CAD build for the part. Positions are in the model's coordinates, mm. Coordinates: 2 decimals unless noted, no trailing zeros. Loops run counter-clockwise (first coordinate to the right, second up) from the corner with the lowest first, then second, coordinate; pieces in that order, holes last. Notation, with made-up numbers: (70, 52.5) -> (103, 52.5) arc R38 ccw to (103, 91.5) -> close; hole circle Ø10 at (60.25, 56). An arc over 180 degrees is marked (long way). Return JSON: item names as keys, results as strings. Group by question number.
(1) Saw through at C-C on y = -2.5. Write the cut outline in (x, z).
(2) Probe L1, parallel to X at y = 6.5, z = 0; L2, parallel to X at y = 11.25, z = 3.5; L3, parallel to Z at x = 4, y = -5.75. List the from-to ranges inside material, lowest first.
(3) Flat gauge pins, fed straight in: pin 1 Ø3 at (y, z) = (5, 3.5) entering from -X; pin 2 Ø2 at (y, z) = (-4, -4) entering from -X. Where does each tip first touch, or does it go through?
(4) Mould opens along X. For faces 1 (the face through (-1.352, 0.182, 4.292)), 2 (the face through (0.1, -0.17, 6.35)), 3 (the face through (-4, -13, -3)) say: pulls with the +X half, pulls with the -X half, needs draft (parallel to the pull), parting line crosses it, or undercut.
(5) Saw through at B-B on x = 0. Write the cut outline in (y, z).
(6) Saw through at A-A on z = 0. Write the cut outline in (x, y).
```python
from build123d import *

# Parameters (mm, degrees)
CUT_EXTRUDE1_DEPTH      = 16.800158227
CUT_EXTRUDE1_DEPTH_BACK = 16.800158227
SKETCH2_W               = 6.200894729
SKETCH2_H               = 5
SKETCH2_W_2             = 7.80745867


with BuildPart() as part:
    # Sketch1 → Revolve1 (revolve)
    with BuildSketch(Plane.XY, mode=Mode.PRIVATE) as revolve1_sk:
        Polygon((-4.5, 13), (-5.35, 13), (-6.35, 12), (-6.35, -12), (-5.35, -13), (-4.5, -13), align=None)
    revolve(revolve1_sk.sketch.rotate(Axis((0, 18.016627358, 0), (0, -1, 0)), 270), axis=Axis((0, 18.016627358, 0), (0, -1, 0)))

    # Sketch2 → Cut-Extrude1 (cut, two sides: drawn at the far end of the back side and taken through both)
    with BuildSketch(Plane(origin=(0, 0, 0), x_dir=(1, 0, 0), z_dir=(0, 1, 0)).offset(-CUT_EXTRUDE1_DEPTH_BACK)):
        with Locations((-8.937612772, 0)):
            Rectangle(SKETCH2_W, SKETCH2_H)
        with Locations((9.740894743, 0)):
            Rectangle(SKETCH2_W_2, SKETCH2_H)
    extrude(amount=CUT_EXTRUDE1_DEPTH + CUT_EXTRUDE1_DEPTH_BACK, mode=Mode.SUBTRACT)


solid = part.part
```
Geometry results:
{
 "1": {"outline": "(-5.84, -2.5) arc R6.35 ccw to (5.84, -2.5) -> (5.84, 2.5) arc R6.35 ccw to (-5.84, 2.5) -> close; hole circle Ø9 at (0, 0)"},
 "2": {"L1": "-5.84 to -4.5, 4.5 to 5.84", "L2": "-5.3 to -2.83, 2.83 to 5.3", "L3": "-4.93 to -2.06, 2.06 to 4.93"},
 "3": {"pin 1": "x = -5.84", "pin 2": "x = -5.6"},
 "4": {"face 1": "undercut", "face 2": "parting line crosses it", "face 3": "needs draft"},
 "5": {"outline": "(-13, -5.35) -> (-12, -6.35) -> (12, -6.35) -> (13, -5.35) -> (13, -4.5) -> (-13, -4.5) -> close; (-13, 4.5) -> (13, 4.5) -> (13, 5.35) -> (12, 6.35) -> (-12, 6.35) -> (-13, 5.35) -> close"},
 "6": {"outline": "(-5.84, -12.51) -> (-5.35, -13) -> (-4.5, -13) -> (-4.5, 13) -> (-5.35, 13) -> (-5.84, 12.51) -> close; (4.5, -13) -> (5.35, -13) -> (5.84, -12.51) -> (5.84, 12.51) -> (5.35, 13) -> (4.5, 13) -> close"}
}
